Autodesk Inventor part; units mm, degrees
ref_plane "YZ Plane" through (0, 0, 0) normal (1, 0, 0) x (0, 1, 0)
ref_plane "XZ Plane" through (0, 0, 0) normal (0, 1, 0) x (-1, 0, 0)
ref_plane "XY Plane" through (0, 0, 0) normal (0, 0, 1) x (1, 0, 0)
sketch "Sketch1" plane through (0, 0, 0) normal (0, 0, 1) x (1, 0, 0)
  circle A0 centre (-5.0359, -76.6135) radius 1.1
  line L0 (-5.0359, -76.6135) -> (-5.0359, -51.6135) construction
  line L1 (-36.2859, -51.6135) -> (26.2141, -51.6135) construction
  line L2 (26.2141, -51.6135) -> (26.2141, -101.6135) construction
  line L3 (26.2141, -101.6135) -> (-36.2859, -101.6135) construction
  line L4 (-36.2859, -101.6135) -> (-36.2859, -51.6135) construction
  line L5 (-5.0359, -76.6135) -> (26.2141, -76.6135) construction
  line L6 (2.9641, -58.0535) -> (-19.6359, -58.0535)
  line L7 (-19.6359, -58.0535) -> (-19.6359, -60.8035)
  line L8 (-19.6359, -60.8035) -> (-12.7609, -60.8035)
  line L9 (-12.7609, -60.8035) -> (-12.7609, -62.6285)
  line L10 (-12.7609, -62.6285) -> (-19.6359, -62.6285)
  arc A1 (-19.6359, -62.6285) -> (-21.3019, -64.2945) centre (-19.6359, -64.2945) ccw
  line L11 (-19.6359, -60.8035) -> (-19.6359, -62.6285) construction
  line L12 (-21.3019, -66.1595) -> (-21.3019, -64.2945)
  line L13 (-21.3019, -66.1595) -> (-25.3019, -66.1595)
  arc A2 (-25.3019, -66.1595) -> (-26.9679, -67.8255) centre (-25.3019, -67.8255) ccw
  line L14 (-26.9679, -67.8255) -> (-26.9679, -75.6235)
  line L15 (-26.9679, -75.6235) -> (-28.3679, -75.6235)
  line L16 (-28.3679, -75.6235) -> (-28.3679, -67.8235)
  line L17 (-28.3679, -67.8235) -> (-31.7679, -67.8235)
  line L18 (-31.7679, -67.8235) -> (-31.7679, -86.8235)
  line L19 (-31.7679, -86.8235) -> (-28.3679, -86.8235)
  line L20 (-28.3679, -86.8235) -> (-28.3679, -79.0235)
  line L21 (-28.3679, -79.0235) -> (-26.9679, -79.0235)
  line L22 (-26.9679, -79.0235) -> (-26.9679, -86.8235)
  arc A3 (-26.9679, -86.8235) -> (-25.3019, -88.4895) centre (-25.3019, -86.8235) ccw
  line L23 (-25.3019, -88.4895) -> (-20.3359, -88.4895)
  line L24 (-20.3359, -88.4895) -> (-15.8208, -94.536)
  arc A4 (-15.8208, -94.536) -> (-14.6189, -95.1385) centre (-14.6189, -93.6385) ccw
  line L25 (-14.6189, -95.1385) -> (7.1805, -95.1385)
  arc A5 (7.1805, -95.1385) -> (8.784, -93.9247) centre (7.1805, -93.4725) ccw
  line L26 (8.784, -93.9247) -> (10.3101, -88.5135)
  line L27 (10.3101, -88.5135) -> (11.8101, -88.5135)
  line L28 (11.8101, -88.5135) -> (13.5395, -93.9985)
  arc A6 (13.5395, -93.9985) -> (15.1284, -95.1635) centre (15.1284, -93.4975) ccw
  line L29 (15.1284, -95.1635) -> (19.0084, -95.1635)
  arc A7 (19.0084, -95.1635) -> (20.6518, -93.771) centre (19.0084, -93.4975) ccw
  arc A8 (20.6518, -93.771) -> (20.6518, -67.5009) centre (-58.2626, -80.636) ccw
  line L30 (20.6518, -93.771) -> (20.6518, -67.5009) construction
  arc A9 (20.6518, -67.5009) -> (19.0143, -66.1135) centre (19.0143, -67.7735) ccw
  line L31 (19.0143, -66.1135) -> (15.1343, -66.1135)
  arc A10 (15.1343, -66.1135) -> (13.5454, -67.2785) centre (15.1343, -67.7795) ccw
  line L32 (13.5454, -67.2785) -> (11.816, -72.7635)
  line L33 (11.816, -72.7635) -> (10.316, -72.7635)
  line L34 (10.316, -72.7635) -> (8.7969, -67.3773)
  line L35 (2.9641, -58.0535) -> (3.0391, -58.0535)
  line L36 (3.0391, -58.0535) -> (3.0391, -60.8035)
  line L37 (3.0391, -60.8035) -> (-3.1109, -60.8035)
  line L38 (-3.1109, -60.8035) -> (-3.1109, -62.6285)
  line L39 (-3.1109, -62.6285) -> (3.0541, -62.6285)
  arc A11 (4.7141, -64.2885) -> (3.0541, -62.6285) centre (3.0541, -64.2885) ccw
  line L40 (4.7141, -64.2885) -> (4.7141, -66.1635)
  line L41 (4.7141, -66.1635) -> (7.1935, -66.1635)
  arc A12 (8.7969, -67.3773) -> (7.1935, -66.1635) centre (7.1935, -67.8295) ccw
  arc A13 (17.4947, -91.7285) -> (17.4954, -69.5485) centre (-58.2626, -80.636) ccw
  line L42 (17.4947, -91.7285) -> (16.4255, -91.7285)
  line L43 (16.4255, -91.7285) -> (14.3287, -85.0785)
  line L44 (14.3287, -85.0785) -> (7.7099, -85.0785)
  line L45 (7.7099, -85.0785) -> (5.8414, -91.7035)
  line L46 (5.8414, -91.7035) -> (-13.6489, -91.7035)
  line L47 (-13.6489, -91.7035) -> (-18.6139, -85.0545)
  line L48 (-18.6139, -85.0545) -> (-23.5329, -85.0545)
  line L49 (-23.5329, -85.0545) -> (-23.5329, -76.6135)
  line L50 (-23.5329, -76.6135) -> (-23.5329, -69.5945)
  line L51 (-23.5329, -69.5945) -> (-17.8669, -69.5945)
  line L52 (-17.8669, -69.5945) -> (-17.8669, -66.0635)
  line L53 (-17.8669, -66.0635) -> (-9.3259, -66.0635)
  line L54 (-9.3259, -66.0635) -> (-9.3259, -61.4885)
  line L55 (-9.3259, -61.4885) -> (-6.5459, -61.4885)
  line L56 (-6.5459, -61.4885) -> (-6.5459, -66.0635)
  line L57 (-6.5459, -66.0635) -> (1.2791, -66.0635)
  line L58 (1.2791, -66.0635) -> (1.2791, -69.5985)
  line L59 (1.2791, -69.5985) -> (5.8544, -69.5985)
  line L60 (5.8544, -69.5985) -> (7.7158, -76.1985)
  line L61 (7.7158, -76.1985) -> (14.3346, -76.1985)
  line L62 (14.3346, -76.1985) -> (16.4314, -69.5485)
  line L63 (16.4314, -69.5485) -> (17.4954, -69.5485)
  line L64 (-23.5329, -76.6135) -> (-5.0359, -76.6135) construction
  line L65 (-6.5459, -66.0635) -> (-9.3259, -66.0635)
  arc A14 (13.0515, -76.1985) -> (14.7205, -74.9747) centre (13.0515, -74.4485) ccw
  arc A15 (7.3562, -74.9235) -> (9.0405, -76.1985) centre (9.0405, -74.4485) ccw
  arc A16 (14.7146, -86.3022) -> (13.0456, -85.0785) centre (13.0456, -86.8285) ccw
  arc A17 (9.0346, -85.0785) -> (7.3503, -86.3535) centre (9.0346, -86.8285) ccw
  arc A18 (1.2791, -67.8485) -> (3.0291, -69.5985) centre (3.0291, -67.8485) ccw
  arc A19 (-19.6169, -69.5945) -> (-17.8669, -67.8445) centre (-19.6169, -67.8445) ccw
  arc A20 (-18.089, -85.7574) -> (-19.4912, -85.0545) centre (-19.4912, -86.8045) ccw
  point P0 (0, 0)
  dimension "d9" = 50
  dimension "d22" = 18.56
  dimension "d23" = 8
  dimension "d24" = 22.6
  dimension "d26" = 2.75
  dimension "d27" = 6.875
  dimension "d28" = 1.825
  dimension "d31" = 3.531
  dimension "d32" = 1.666
  dimension "d33" = 1.666
  dimension "d34" = 1.666
  dimension "d40" = 4
  dimension "d42" = 0.99
  dimension "d43" = 1.4
  dimension "d44" = 3.4
  dimension "d45" = 7.8
  dimension "d46" = 19
  dimension "d47" = 1.666
  dimension "d55" = 15.3
  dimension "d56" = 53.25
  dimension "d58" = 18.525
  dimension "d62" = 1.5
  dimension "d65" = 105.75
  dimension "d66" = 18
  dimension "d67" = 1.666
  dimension "d68" = 11.9
  dimension "d69" = 107.5
  dimension "d70" = 1.5
  dimension "d72" = 18.55
  dimension "d73" = 1.666
  dimension "d75" = 1.666
  dimension "d77" = 3.88
  dimension "d78" = 80
  dimension "d82" = 1.66
  dimension "d85" = 10.5
  dimension "d87" = 3.88
  dimension "d88" = 15.75
  dimension "d90" = 107.5
  dimension "d91" = 105.75
  dimension "d94" = 0.075
  dimension "d95" = 6.15
  dimension "d96" = 1.66
  dimension "d97" = 1.666
  dimension "d98" = 9.75
  dimension "d99" = 10.45
  dimension "d101" = 10.55
  dimension "d107" = 3.5
  dimension "d108" = 3.5
  dimension "d111" = 3.5
  dimension "d112" = 3.5
  dimension "d113" = 3.5
  dimension "d114" = 3.5
  dimension "d116" = 3.5
extrude "Extrusion1" add sketch "Sketch1" along normal blind 2 contours L35 L36 L37 L38 L39 A11 L40 L41 A12 L34 L33 L32 A10 L31 A9 A8 A7 L29 A6 L28 L27 L26 A5 L25 A4 L24 L23 A3 L22 L21 L20 L19 L18 L17 L16 L15 L14 A2 L13 L12 A1 L10 L9 L8 L7 L6 | L65 L54 L55 L56
sketch "Sketch2" plane through (0, 0, 0) normal (0, 0, -1) x (-1, 0, 0)
  line L0 (-23.7374, -56.0535) -> (33.7679, -56.0535)
  line L1 (33.7679, -56.0535) -> (33.7679, -97.1385)
  line L2 (33.7679, -97.1385) -> (-23.7374, -97.1385)
  line L3 (-23.7374, -97.1385) -> (-23.7374, -56.0535)
  arc A0 (-23.7374, -56.0535) -> (-23.7374, -97.1385) centre (16.3001, -76.596) ccw
  line L4 (-3.0391, -58.0535) -> (19.6359, -58.0535) construction
  line L5 (-3.0391, -60.8035) -> (-3.0391, -58.0535) construction
  line L6 (3.1109, -60.8035) -> (-3.0391, -60.8035) construction
  line L7 (3.1109, -62.6285) -> (3.1109, -60.8035) construction
  line L8 (-3.0541, -62.6285) -> (3.1109, -62.6285) construction
  arc A1 (-3.0541, -62.6285) -> (-4.7141, -64.2885) centre (-3.0541, -64.2885) ccw construction
  line L9 (-4.7141, -66.1635) -> (-4.7141, -64.2885) construction
  line L10 (-7.1935, -66.1635) -> (-4.7141, -66.1635) construction
  arc A2 (-7.1935, -66.1635) -> (-8.7969, -67.3773) centre (-7.1935, -67.8295) ccw construction
  line L11 (-10.316, -72.7635) -> (-8.7969, -67.3773) construction
  line L12 (-11.816, -72.7635) -> (-10.316, -72.7635) construction
  line L13 (-13.5454, -67.2785) -> (-11.816, -72.7635) construction
  arc A3 (-13.5454, -67.2785) -> (-15.1343, -66.1135) centre (-15.1343, -67.7795) ccw construction
  line L14 (-19.0143, -66.1135) -> (-15.1343, -66.1135) construction
  arc A4 (-19.0143, -66.1135) -> (-20.6518, -67.5009) centre (-19.0143, -67.7735) ccw construction
  arc A5 (-20.6518, -67.5009) -> (-20.6518, -93.771) centre (58.2626, -80.636) ccw construction
  arc A6 (-20.6518, -93.771) -> (-19.0084, -95.1635) centre (-19.0084, -93.4975) ccw construction
  line L15 (-15.1284, -95.1635) -> (-19.0084, -95.1635) construction
  arc A7 (-15.1284, -95.1635) -> (-13.5395, -93.9985) centre (-15.1284, -93.4975) ccw construction
  line L16 (-11.8101, -88.5135) -> (-13.5395, -93.9985) construction
  line L17 (-10.3101, -88.5135) -> (-11.8101, -88.5135) construction
  line L18 (-8.784, -93.9247) -> (-10.3101, -88.5135) construction
  arc A8 (-8.784, -93.9247) -> (-7.1805, -95.1385) centre (-7.1805, -93.4725) ccw construction
  line L19 (14.6189, -95.1385) -> (-7.1805, -95.1385) construction
  arc A9 (14.6189, -95.1385) -> (15.8208, -94.536) centre (14.6189, -93.6385) ccw construction
  line L20 (20.3359, -88.4895) -> (15.8208, -94.536) construction
  line L21 (25.3019, -88.4895) -> (20.3359, -88.4895) construction
  arc A10 (25.3019, -88.4895) -> (26.9679, -86.8235) centre (25.3019, -86.8235) ccw construction
  line L22 (26.9679, -79.0235) -> (26.9679, -86.8235) construction
  line L23 (28.3679, -79.0235) -> (26.9679, -79.0235) construction
  line L24 (28.3679, -86.8235) -> (28.3679, -79.0235) construction
  line L25 (31.7679, -86.8235) -> (28.3679, -86.8235) construction
  line L26 (31.7679, -67.8235) -> (31.7679, -86.8235) construction
  line L27 (28.3679, -67.8235) -> (31.7679, -67.8235) construction
  line L28 (28.3679, -75.6235) -> (28.3679, -67.8235) construction
  line L29 (26.9679, -75.6235) -> (28.3679, -75.6235) construction
  line L30 (26.9679, -67.8255) -> (26.9679, -75.6235) construction
  arc A11 (26.9679, -67.8255) -> (25.3019, -66.1595) centre (25.3019, -67.8255) ccw construction
  line L31 (21.3019, -66.1595) -> (25.3019, -66.1595) construction
  line L32 (21.3019, -64.2945) -> (21.3019, -66.1595) construction
  arc A12 (21.3019, -64.2945) -> (19.6359, -62.6285) centre (19.6359, -64.2945) ccw construction
  line L33 (12.7609, -62.6285) -> (19.6359, -62.6285) construction
  line L34 (12.7609, -60.8035) -> (12.7609, -62.6285) construction
  line L35 (19.6359, -60.8035) -> (12.7609, -60.8035) construction
  line L36 (19.6359, -58.0535) -> (19.6359, -60.8035) construction
  line L37 (-17.4947, -91.7285) -> (-16.4255, -91.7285) construction
  arc A13 (-17.4954, -69.5485) -> (-17.4947, -91.7285) centre (58.2626, -80.636) ccw construction
  line L38 (-16.4314, -69.5485) -> (-17.4954, -69.5485) construction
  line L39 (-14.7205, -74.9747) -> (-16.4314, -69.5485) construction
  arc A14 (-14.7205, -74.9747) -> (-13.0515, -76.1985) centre (-13.0515, -74.4485) ccw construction
  line L40 (-9.0405, -76.1985) -> (-13.0515, -76.1985) construction
  arc A15 (-9.0405, -76.1985) -> (-7.3562, -74.9235) centre (-9.0405, -74.4485) ccw construction
  line L41 (-5.8544, -69.5985) -> (-7.3562, -74.9235) construction
  line L42 (-3.0291, -69.5985) -> (-5.8544, -69.5985) construction
  arc A16 (-3.0291, -69.5985) -> (-1.2791, -67.8485) centre (-3.0291, -67.8485) ccw construction
  line L43 (-1.2791, -66.0635) -> (-1.2791, -67.8485) construction
  line L44 (17.8669, -66.0635) -> (-1.2791, -66.0635) construction
  line L45 (17.8669, -67.8445) -> (17.8669, -66.0635) construction
  arc A17 (17.8669, -67.8445) -> (19.6169, -69.5945) centre (19.6169, -67.8445) ccw construction
  line L46 (23.5329, -69.5945) -> (19.6169, -69.5945) construction
  line L47 (23.5329, -85.0545) -> (23.5329, -69.5945) construction
  line L48 (19.4912, -85.0545) -> (23.5329, -85.0545) construction
  arc A18 (19.4912, -85.0545) -> (18.089, -85.7574) centre (19.4912, -86.8045) ccw construction
  line L49 (13.6489, -91.7035) -> (18.089, -85.7574) construction
  line L50 (-5.8414, -91.7035) -> (13.6489, -91.7035) construction
  line L51 (-7.3503, -86.3535) -> (-5.8414, -91.7035) construction
  arc A19 (-7.3503, -86.3535) -> (-9.0346, -85.0785) centre (-9.0346, -86.8285) ccw construction
  line L52 (-13.0456, -85.0785) -> (-9.0346, -85.0785) construction
  arc A20 (-13.0456, -85.0785) -> (-14.7146, -86.3022) centre (-13.0456, -86.8285) ccw construction
  line L53 (-16.4255, -91.7285) -> (-14.7146, -86.3022) construction
  arc A21 (-20.6518, -67.5009) -> (-20.6518, -93.771) centre (58.2626, -80.636) ccw construction
  line L54 (-21.7374, -80.636) -> (-18.3024, -80.6385) construction
  line L55 (16.3001, -76.596) -> (-28.6999, -76.596) construction
  line L56 (5.0152, -56.0535) -> (5.0152, -97.1385) construction
  arc A22 (33.7679, -97.1385) -> (33.7679, -56.0535) centre (-6.2696, -76.596) ccw
  circle A23 centre (5.0359, -76.6135) radius 1.1
  point P0 (0, 0)
  dimension "d119" = 2
  dimension "d120" = 2
  dimension "d121" = 2
  dimension "d122" = 2
  dimension "d123" = 45
extrude "Extrusion2" add sketch "Sketch2" against normal blind 1
fillet "Fillet1" radius 10 4 edges at (23.7374, -97.1385, 0.5) (23.7374, -56.0535, 0.5) (-33.7679, -56.0535, 0.5) (-33.7679, -97.1385, 0.5)
properties part number "engine _light"
Read the model definition and answer for the solid it produces. Units are mm, in the model's axes. A direction names the side the tool comes from. Give positions to 0.01 mm unless a question says otherwise; leave off trailing zeros. Write each loop counter-clockwise with the first axis right and the second up, starting at its lowest first coordinate (ties: lowest second). Pieces come first, ordered by that corner, then holes. Notation, with made-up numbers: (-25, -5) - (18, -5) arc R25 cw to (18, 12) - close; hole circle Ø9 at (59, 42). An arc over 180 degrees is marked (long way). Answer in a Markdown table with one row per item. Add a question column.
Item 1: Find the intervals of material crossed by L1, parallel to Y at x = -6, z = 1.3; L2, parallel to X at y = -72, z = 1.3; L3, parallel to Y at x = -22.5, z = 1.75, in increasing order.
Item 2: Section A-A, the plane x = -24.5 is taken. Write down the section's boundary in (y, z).
Item 3: A tool of negligible diameter and unlimited length cuts with its end or side. For faces 1 (the face through (-20.8, -63.1, 1.5)), 2 (the face through (-18.11, -91.47, 1.49)), 3 (the face through (12.693, -69.983, 1.493)), 4 (the face through (22.91, -95.26, 0.51)), 5 (the face through (-18.4, -69.1, 1.5)), from which of +Z, -Z, +X, -X, +Y, -Y can it reach the whole face along a straight path? Write none if from no direction.
Item 4: Determine the mould class of faces 6 (the face through (8.2, -94.79, 1.49)), 7 (the face through (6.606, -88.991, 1.493)), 8 (the face through (28.7, -76.4, 0.5)), 9 (the face through (23.056, -58.04, 0.507)) for opening direction Y: pulls with the +Y half, pulls with the -Y half, needs draft (parallel to the pull), parting line crosses it, or undercut.
Item 5: Flat-ended cylindrical pins translate along their axes: P1, Ø12, axis at x = -0.5, y = -87, coming from the +Z side; P2, Ø1.1, axis at x = -29.5, z = 1.5, coming from the +Y side; P3, Ø5, axis at x = 18, y = -63, coming from the +Z side; P4, Ø0.8, axis at x = -23, z = 1.5, coming from the -Y side. Find the tip coordinate at first contact, or state that the pin passes through.
Item 6: Section D-D, the plane x = -11.5 is taken. Write down the section's boundary in (y, z).
Item 7: Section B-B, the plane y = -59 is taken. Write down the section's boundary in (x, z).
Item 8: Section C-C, the plane z = 0.4 is taken. Write down the section's boundary in (x, y), and give its area (3 significant figures).
Recorded:
| question | item | result |
|---|---|---|
| 1 | L1 | y = -95.14 to -91.7, -66.06 to -58.05 |
| 1 | L2 | x = -31.77 to -28.37, -26.97 to -23.53, 6.53 to 10.1, 12.06 to 15.66, 17.81 to 21.27 |
| 1 | L3 | y = -88.49 to -85.05, -69.59 to -66.16 |
| 2 | outline | (-97.14, 0) - (-56.05, 0) - (-56.05, 1) - (-66.16, 1) - (-66.16, 2) - (-88.49, 2) - (-88.49, 1) - (-97.14, 1) - close |
| 3 | face 1 | +Z, -X, +Y |
| 3 | face 2 | +Z, -X, -Y |
| 3 | face 3 | +Z, +Y |
| 3 | face 4 | +Z, -Z, +X, -Y |
| 3 | face 5 | +Z |
| 4 | face 6 | pulls with the -Y half |
| 4 | face 7 | undercut |
| 4 | face 8 | parting line crosses it |
| 4 | face 9 | pulls with the +Y half |
| 5 | P1 | stops at z = 2 |
| 5 | P2 | stops at y = -56.29 |
| 5 | P3 | stops at z = 1 |
| 5 | P4 | stops at y = -88.49 |
| 6 | outline | (-97.14, 0) - (-56.05, 0) - (-56.05, 1) - (-58.05, 1) - (-58.05, 2) - (-66.06, 2) - (-66.06, 1) - (-91.7, 1) - (-91.7, 2) - (-95.14, 2) - (-95.14, 1) - (-97.14, 1) - close |
| 7 | outline | (-34.19, 0) - (24.16, 0) - (24.16, 1) - (3.04, 1) - (3.04, 2) - (-19.64, 2) - (-19.64, 1) - (-34.19, 1) - close |
| 8 | outline | (-36.64, -90.15) arc R10 ccw to (-27.1, -97.14) - (17.07, -97.14) arc R10 ccw to (26.61, -90.15) arc R45 ccw to (26.61, -63.04) arc R10 ccw to (17.07, -56.05) - (-27.1, -56.05) arc R10 ccw to (-36.64, -63.04) arc R45 ccw to start; hole circle Ø2.2 at (-5.04, -76.61) |
| 8 | area | 2,600 mm2 |
